from build123d import *

# Parameters (mm, degrees)
SKETCH9_R           = 195.99424204
SKETCH9_R_2         = 171.779053358
BOSS_EXTRUDE1_DEPTH = 280.985470498
CHAMFER1_SIZE       = 10


with BuildPart() as part:
    # Sketch4 → Revolve3 (revolve)
    with BuildSketch(Plane.XY, mode=Mode.PRIVATE) as revolve3_sk:
        Polygon((-253.775337615, -190), (-245.99424204, -190), (-245.99424204, -150), (-235.99424204, -150), (-235.99424204, -100), (-225.99424204, -100), (-225.99424204, -50), (-215.99424204, -50), (-215.99424204, 0), (-205.99424204, 0), (-205.99424204, 50), (-195.99424204, 50), (-195.99424204, 110), (-205.99424204, 110), (-205.99424204, 60), (-215.99424204, 60), (-215.99424204, 10), (-225.99424204, 10), (-225.99424204, -40), (-235.99424204, -40), (-235.99424204, -90), (-245.99424204, -90), (-245.99424204, -140), (-253.775337615, -140), align=None)
    revolve(revolve3_sk.sketch.rotate(Axis((0, 105.494376543, 0), (0, -1, 0)), 270), axis=Axis((0, 105.494376543, 0), (0, -1, 0)))

    # Sketch9 → Boss-Extrude1 (add)
    with BuildSketch(Plane(origin=(0, 110, 0), x_dir=(1, 0, 0), z_dir=(0, 1, 0))):
        with Locations(Location((0, 0, 0), (0, 0, 270))):
            Circle(SKETCH9_R)
        with Locations(Location((0, 0, 0), (0, 0, 270))):
            Circle(SKETCH9_R_2, mode=Mode.SUBTRACT)
    extrude(amount=-BOSS_EXTRUDE1_DEPTH)

    # Chamfer1
    chamfer1_edges = [part.edges().sort_by_distance(p)[0] for p in [
        (0, -170.985470498, -195.99424204),
    ]]
    chamfer(chamfer1_edges, length=CHAMFER1_SIZE)


solid = part.part
CAD build for the part. Positions are in the model's coordinates, mm. A direction names the side the tool comes from. Round coordinates to 2 decimals unless told otherwise and drop trailing zeros. Write each loop counter-clockwise with the first axis right and the second up, starting at its lowest first coordinate (ties: lowest second). Pieces come first, ordered by that corner, then holes. Notation, with made-up numbers: (-40, 58.5) -> (-10, 58.5) arc R19 ccw to (-10, 68.5) -> close; hole circle Ø10 at (30.25, -5). An arc over 180 degrees is marked (long way). Answer as a JSON object with one key per item and string values.
(1) Pin check, flat tips, straight feed: P1, Ø1, axis at y = -95, z = -137, coming from the +X side; P2, Ø1.5, axis at x = -64.5, y = 79, coming from the +Z side; P3, Ø4, axis at x = 193.5, z = -28, coming from the -Y side. Stop position of each tip, or through.
Reported:
{"P1": "stops at x = 204.65", "P2": "stops at z = 195.88", "P3": "stops at y = -163.46"}
(2) Probe probe 1 along X at (y, z) = (-83, 0); probe 2 along X at (y, z) = (43, 0); probe 3 along X at (y, z) = (-179, 0). List the from-to ranges inside material, lowest first. Write a range as [from, to].
Reported:
{"probe 1": "x = [-235.99, -225.99], [-195.99, -171.78], [171.78, 195.99], [225.99, 235.99]", "probe 2": "x = [-215.99, -205.99], [-195.99, -171.78], [171.78, 195.99], [205.99, 215.99]", "probe 3": "x = [-253.78, -245.99], [245.99, 253.78]"}
(3) Two-plate mould, pull along Z, no slides. Class faces 1 (the face through (-167.694, -28.526, -37.238)), 2 (the face through (125.344, 84.65, -163.47)), 3 (the face through (121.3, -40, -191.2)): +Z half, -Z half, draft (parallel to the pull), parting line (faces both ways), or undercut.
Reported:
{"face 1": "undercut", "face 2": "parting line", "face 3": "draft"}
(4) Band-saw the part on A-A, the plane y = 20. List the corners of the cut face in (x, z), then the cut area to 3 significant figures.
Reported:
{"outline": "circle Ø431.99 at (0, 0); circle Ø391.99 at (0, 0); hole circle Ø411.99 at (0, 0); hole circle Ø343.56 at (0, 0)", "area": "41,200 mm^2"}
(5) Band-saw the part on B-B, the plane y = -127.5. List the corners of the cut face in (x, z).
Reported:
{"outline": "circle Ø491.99 at (0, 0); circle Ø391.99 at (0, 0); hole circle Ø471.99 at (0, 0); hole circle Ø343.56 at (0, 0)"}
(6) Which spindle directions (+Z, -Z, +X, -X, +Y, -Y) get a long thin tool onto all of the face, cutting with end or side? Do faces 4 (the face through (236, -90, -17)), 5 (the face through (-191.334, -54.016, -42.488)). Say none if no direction does.
Reported:
{"face 4": "+Y", "face 5": "-Y"}
